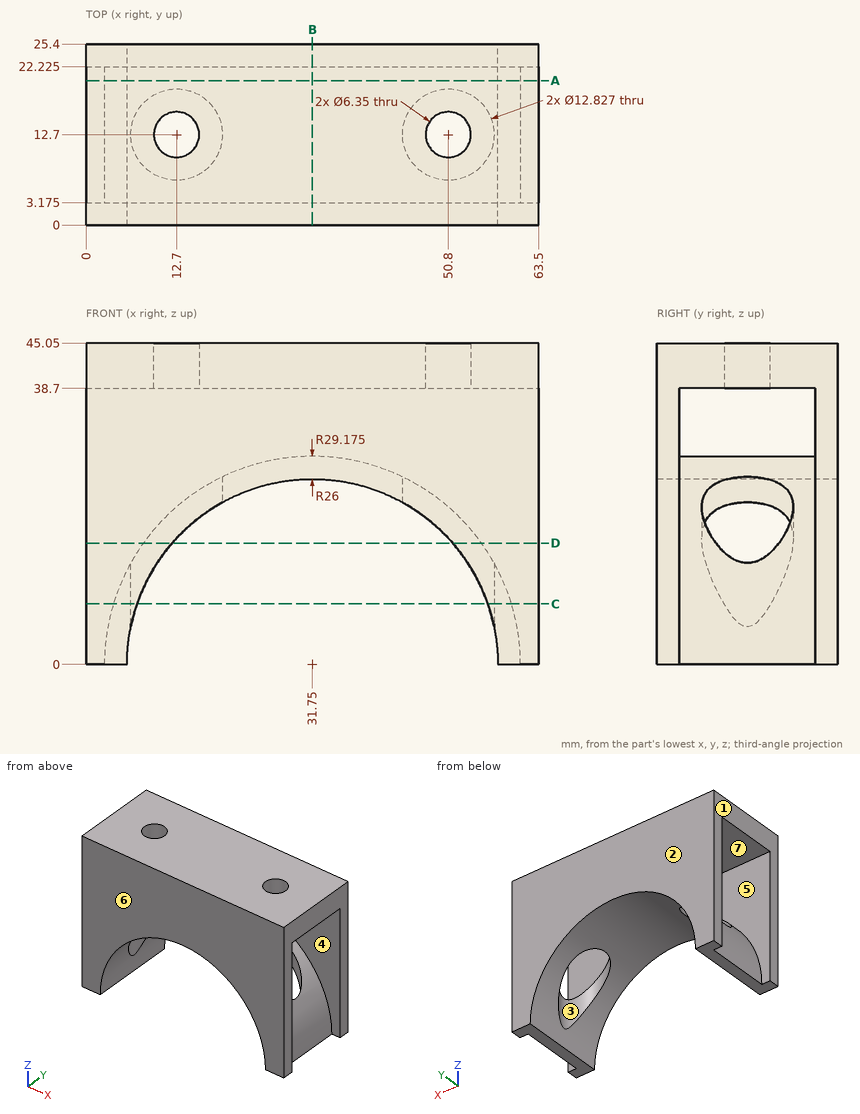
Job drawing, mm, ordinate dimensions from the low corner. One solid piece. A direction names the side the tool comes from. Round coordinates to 2 decimals unless told otherwise and drop trailing zeros. Loops run counter-clockwise (first coordinate to the right, second up) from the corner with the lowest first, then second, coordinate; pieces in that order, holes last. Notation, with made-up numbers: (-6.5, 62.25) -> (14.5, 62.25) arc R18 cw to (14.5, 76.25) -> close; hole circle Ø6 at (-0.5, 51.25). An arc over 180 degrees is marked (long way). Use a Markdown table: item, result.
1) Cut at D-D, the plane z = 17. List the corners of the cut face in (x, y) (1 decimal), and give its area (3 significant figures).
The answers:
| item | result |
|---|---|
| outline | (0, 0) -> (12.1, 0) -> (12.1, 6.3) arc R6.4 cw to (8, 8.3) -> (8, 3.2) -> (0, 3.2) -> close; (0, 22.2) -> (8, 22.2) -> (8, 17.1) arc R6.4 cw to (12.1, 19.1) -> (12.1, 25.4) -> (0, 25.4) -> close; (51.4, 0) -> (63.5, 0) -> (63.5, 3.2) -> (55.5, 3.2) -> (55.5, 8.3) arc R6.4 cw to (51.4, 6.3) -> close; (51.4, 19.1) arc R6.4 cw to (55.5, 17.1) -> (55.5, 22.2) -> (63.5, 22.2) -> (63.5, 25.4) -> (51.4, 25.4) -> close |
| area | 215 mm2 |
2) Cut at A-A, the plane y = 20.25. List the corners of the cut face in (x, z) (3 decimals).
The answers:
| item | result |
|---|---|
| outline | (0, 38.7) -> (63.5, 38.7) -> (63.5, 45.05) -> (0, 45.05) -> close; (2.575, 0) -> (5.75, 0) arc R26 cw to (57.75, 0) -> (60.925, 0) arc R29.175 ccw to start |
3) Tool access for the marked faces 5, 6 and 7: list every direction of +Z, -Z, +X, -X, +Y, -Y with a clear straight run to the whole face (end or side of a thin tool).
The answers:
| item | result |
|---|---|
| face 5 | none |
| face 6 | +Z, -Z, +X, -X, -Y |
| face 7 | +X, -X |
4) Pull direction Y, two halves, no side cores. Call the marked faces 1, 2, 3 and 4: pulls with the +Y half, pulls with the -Y half, needs draft (parallel to the pull), parting line crosses it, or undercut.
The answers:
| item | result |
|---|---|
| face 1 | needs draft |
| face 2 | pulls with the +Y half |
| face 3 | undercut |
| face 4 | undercut |
5) Cut at C-C, the plane z = 8.5. List the corners of the cut face in (x, y) (1 decimal), and give its area (3 significant figures).
The answers:
| item | result |
|---|---|
| outline | (0, 0) -> (7.2, 0) -> (7.2, 9.4) arc R6.4 cw to (7.2, 16) -> (7.2, 25.4) -> (0, 25.4) -> (0, 22.2) -> (3.8, 22.2) -> (3.8, 3.2) -> (0, 3.2) -> close; (56.3, 0) -> (63.5, 0) -> (63.5, 3.2) -> (59.7, 3.2) -> (59.7, 22.2) -> (63.5, 22.2) -> (63.5, 25.4) -> (56.3, 25.4) -> (56.3, 16) arc R6.4 cw to (56.3, 9.4) -> close |
| area | 210 mm2 |
6) Cut at B-B, the plane x = 31.75. List the corners of the cut face in (y, z) (3 decimals).
The answers:
| item | result |
|---|---|
| outline | (0, 26) -> (25.4, 26) -> (25.4, 45.05) -> (0, 45.05) -> close; hole (3.175, 29.175) -> (22.225, 29.175) -> (22.225, 38.7) -> (3.175, 38.7) -> close |
7) Drop flat-ended pins along their axis: pin 1 Ø15 at (x, y) = (17, 16) entering from -Z; pin 2 Ø5.5 at (x, y) = (50.8, 12.7) entering from -Z; pin 3 Ø3 at (y, z) = (15.5, 25.5) entering from +X. Give the stop position or say it passes through.
The answers:
| item | result |
|---|---|
| pin 1 | stops at z = 14.13 |
| pin 2 | passes through |
| pin 3 | stops at x = 46.04 |
8) Probe line 1 (Y direction, x = 50.8, z = 43) (3 decimals); line 2 (Y direction, x = 39.5, z = 38) (3 decimals); line 3 (X direction, y = 20.5, z = 23.5). List the from-to ranges inside material, lowest first. Write a range as [from, to].
The answers:
| item | result |
|---|---|
| line 1 | y = [0, 9.525], [15.875, 25.4] |
| line 2 | y = [0, 3.175], [22.225, 25.4] |
| line 3 | x = [14.46, 20.63], [42.87, 49.04] |
